Read the model definition and answer for the solid it produces. Units are mm, in the model's axes. Face numbers are marked on the shaded views. Round coordinates to 2 decimals unless told otherwise and drop trailing zeros. Order: outer loops, then holes, each group sorted by start corner. A loop starts at its lowest first (then second) coordinate and runs counter-clockwise, first axis right, second up. Notation, with made-up numbers: (18.5, 81) -> (22.5, 81) arc R11 cw to (22.5, 93) -> close; hole circle Ø3 at (19.25, -21). An arc over 180 degrees is marked (long way). Use a Markdown table: item, result. Add a question column.
1. Section B-B, the plane y = 0 is taken. Give the vertices of the cut face in (x, z).
2. Section C-C, the plane z = 12.5 is taken. Give the vertices of the cut face in (x, y), then the cut area to 3 significant figures.
3. The mould has two halves that part along Y. Classify the marked faces 1, 2 and 3: +Y half, -Y half, draft (parallel to the pull), parting line (faces both ways), or undercut.
4. Section A-A, the plane x = 0 is taken. Give the vertices of the cut face in (y, z).
5. Given pin 1 (8 mm diameter, centred on x = 60, z = 23.5, fed in from -Y); pin 2 (8 mm diameter, centred on x = 60, z = 17, fed in from +Y); pin 3 (4 mm diameter, centred on y = 59.5, z = 20, fed in from +X), each flat-ended and moving along its own axis, determine where each tip first touches the part or whether it passes through.
6. Consider L1, parallel to Y at x = 0, z = 21.5; L2, parallel to X at y = 1, z = 32 (3 decimals); L3, parallel to Z at x = -39.5, y = 14.5. Determine where each line is inside the solid, lowest interval first. Write a range as [from, to].
7. Section D-D, the plane y = 57 is taken. Give the vertices of the cut face in (x, z), then the cut area to 3 significant figures.
```python
from build123d import *

# Parameters (mm, degrees)
SKETCH1_R           = 100
BOSS_EXTRUDE1_DEPTH = 36
SKETCH2_R           = 97
CUT_EXTRUDE2_DEPTH  = 33
SKETCH3_R           = 1.75
SKETCH3_R_2         = 7
SKETCH3_W           = 10
SKETCH3_H           = 14
CUT_EXTRUDE4_DEPTH  = 4


with BuildPart() as part:
    # Sketch1 → Boss-Extrude1 (new body)
    with BuildSketch(Plane.XY):
        Circle(SKETCH1_R)
    extrude(amount=BOSS_EXTRUDE1_DEPTH)

    # Sketch2 → Cut-Extrude2 (cut)
    with BuildSketch(Plane.XY):
        Circle(SKETCH2_R)
    extrude(amount=CUT_EXTRUDE2_DEPTH, mode=Mode.SUBTRACT)

    # Sketch3 → Cut-Extrude4 (cut)
    with BuildSketch(Plane.XY):
        with Locations((110, 24.75)):
            Circle(SKETCH3_R)
        with Locations((110, -24.75)):
            Circle(SKETCH3_R)
        with Locations((110, 0)):
            Circle(SKETCH3_R_2)
        with Locations((-93, 0)):
            Rectangle(SKETCH3_W, SKETCH3_H)
    extrude(amount=CUT_EXTRUDE4_DEPTH, mode=Mode.SUBTRACT)


solid = part.part
```
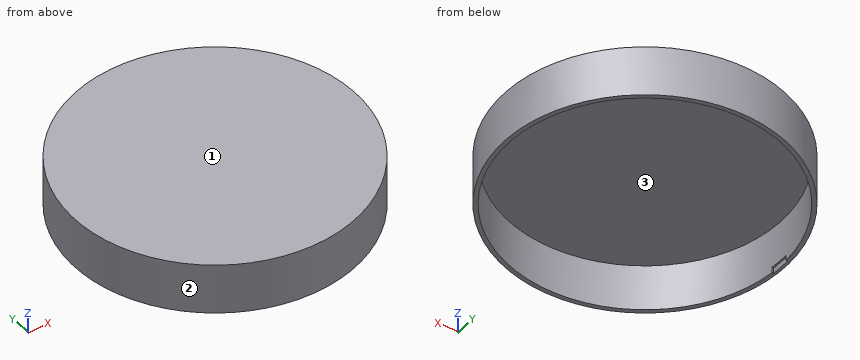
Verdict:
| question | item | result |
|---|---|---|
| 1 | outline | (-100, 0) -> (-98, 0) -> (-98, 4) -> (-97, 4) -> (-97, 33) -> (97, 33) -> (97, 0) -> (100, 0) -> (100, 36) -> (-100, 36) -> close |
| 2 | outline | circle Ø200 at (0, 0); hole circle Ø194 at (0, 0) |
| 2 | area | 1,860 mm2 |
| 3 | face 1 | draft |
| 3 | face 2 | parting line |
| 3 | face 3 | undercut |
| 4 | outline | (-100, 0) -> (-97, 0) -> (-97, 33) -> (97, 33) -> (97, 0) -> (100, 0) -> (100, 36) -> (-100, 36) -> close |
| 5 | pin 1 | stops at y = -82.85 |
| 5 | pin 2 | stops at y = 82.85 |
| 5 | pin 3 | stops at x = 81.82 |
| 6 | L1 | y = [-100, -97], [97, 100] |
| 6 | L2 | x = [-99.995, -96.995], [96.995, 99.995] |
| 6 | L3 | z = [33, 36] |
| 7 | outline | (-82.16, 0) -> (-78.49, 0) -> (-78.49, 33) -> (78.49, 33) -> (78.49, 0) -> (82.16, 0) -> (82.16, 36) -> (-82.16, 36) -> close |
| 7 | area | 736 mm2 |
